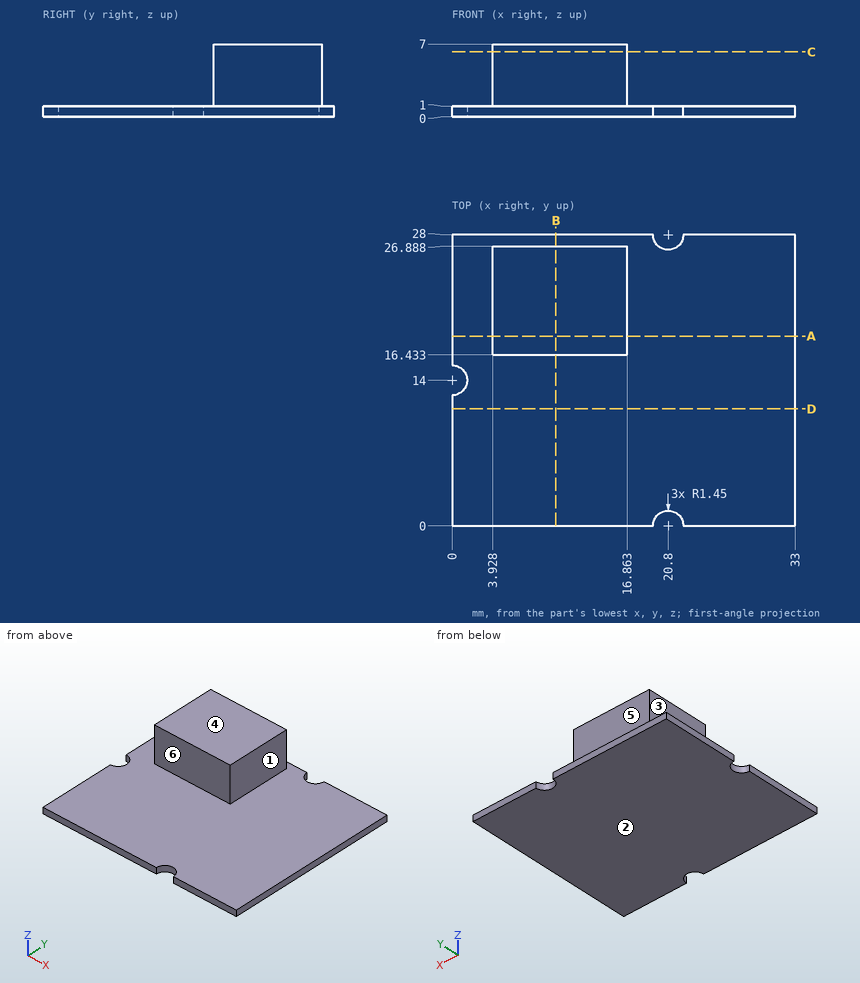
Geometry check sheet. Reference: drawing and pictorial views, mm from the part's lowest x, y, z. A direction names the side the tool comes from. Coordinates: 2 decimals unless noted, no trailing zeros. Write each loop counter-clockwise with the first axis right and the second up, starting at its lowest first coordinate (ties: lowest second). Pieces come first, ordered by that corner, then holes. Notation, with made-up numbers: (38.25, 15) - (82.25, 15) arc R22 ccw to (82.25, 38) - close; hole circle Ø4 at (-24, 31.5). An arc over 180 degrees is marked (long way). One line per question, with ' | ' between items. Start each with the question number.
1. Access from +Z, -Z, +X, -X, +Y, -Y to the whole of each face (thin tool, end or side, straight path). Record for the marked faces 1, 2 and 3.
2. Gauge pin test, flat ends, axial feed: P1, Ø3, axis at x = 13.5, z = 4, coming from the +Y side; P2, Ø1.8, axis at y = 19.5, z = 5.5, coming from the +X side; P3, Ø8.5, axis at x = 8.5, y = 10.5, coming from the +Z side. Record the tip position at first contact, or that the pin passes through.
3. Section check C-C (z = 6.25). Enter the section's corners in (x, y).
4. Section check A-A (y = 18.25). Enter the section's corners in (x, z).
5. Material ranges on line 1 along X through (y, z) = (19.75, 6.25); line 2 along Y through (x, z) = (11, 3.5); line 3 along Z through (x, y) = (4, 11), recorded low to high.
6. Section check D-D (y = 11.25). Enter the section's corners in (x, z).
7. Draft check along Y on the marked faces 4, 5 and 6. Enter one of: released by +Y, released by -Y, zero draft, split by the parting line, or undercut.
8. Section check B-B (x = 10). Enter the section's corners in (y, z).
Computed values:
1) face 1: +Z, +X, +Y, -Y | face 2: -Z, +X, -X, +Y, -Y | face 3: +Z, -X, +Y, -Y
2) P1: y = 26.89 | P2: x = 16.86 | P3: z = 1
3) outline: (3.93, 16.43) - (16.86, 16.43) - (16.86, 26.89) - (3.93, 26.89) - close
4) outline: (0, 0) - (33, 0) - (33, 1) - (16.86, 1) - (16.86, 7) - (3.93, 7) - (3.93, 1) - (0, 1) - close
5) line 1: 3.93 to 16.86 | line 2: 16.43 to 26.89 | line 3: 0 to 1
6) outline: (0, 0) - (33, 0) - (33, 1) - (0, 1) - close
7) face 4: zero draft | face 5: released by +Y | face 6: released by -Y
8) outline: (0, 0) - (28, 0) - (28, 1) - (26.89, 1) - (26.89, 7) - (16.43, 7) - (16.43, 1) - (0, 1) - close
